```python
from build123d import *

# Parameters (mm, degrees)
F0_W     = 254
F0_H     = 101.6
F0_R     = 9.525
F1_DEPTH = 12.7
F2_R     = 6.35
F3_DEPTH = 12.7
F4_R     = 6.35
F5_W     = 0.9328643791
F5_H     = 1.7582587898
F5_W_2   = 0.0005662441
F5_H_2   = 0.0007078052
F6_DEPTH = 254.001


# Not quite as in the source:
# - a feature of the source that left no trace in its solid (it failed there, or was rolled back) is left out


with BuildPart() as f1:
    # F0 (on Front) → F1 (new body)
    with BuildSketch(Plane.XZ):
        with Locations((143.2877514958, 67.8497503132)):
            Rectangle(F0_W, F0_H)
        with Locations((67.0877514958, 67.8497503132)):
            Circle(F0_R, mode=Mode.SUBTRACT)
        with Locations((219.4877514958, 67.8497503132)):
            Circle(F0_R, mode=Mode.SUBTRACT)
    extrude(amount=F1_DEPTH)

    # F2
    f2_edges = [f1.edges().sort_by_distance(p)[0] for p in [
        (16.287751, -6.35, 118.64975),
        (16.287751, -6.35, 17.04975),
        (270.287751, -6.35, 118.64975),
        (270.287751, -6.35, 17.04975),
    ]]
    fillet(f2_edges, radius=F2_R)

    # F0 (on Front) → F3 (join)
    with BuildSketch(Plane.XZ):
        with Locations((143.2877514958, 67.8497503132)):
            Rectangle(F0_W, F0_H)
        with Locations((67.0877514958, 67.8497503132)):
            Circle(F0_R, mode=Mode.SUBTRACT)
        with Locations((219.4877514958, 67.8497503132)):
            Circle(F0_R, mode=Mode.SUBTRACT)
    extrude(amount=F3_DEPTH)

    # F4
    f4_edges = [f1.edges().sort_by_distance(p)[0] for p in [
        (270.287751, -6.35, 118.64975),
        (16.287751, -6.35, 118.64975),
        (270.287751, -6.35, 17.04975),
        (16.287751, -6.35, 17.04975),
    ]]
    fillet(f4_edges, radius=F4_R)

    # F5 (on face) → F6 (cut, through all)
    with BuildSketch(Plane(origin=(16.2877514958, 0, 0), x_dir=(0, -1, 0), z_dir=(-1, 0, 0))):
        with Locations((6.063854089, 49.9223377556)):
            Rectangle(F5_W, F5_H)
        with Locations((8.4549216554, 49.0087680519)):
            Rectangle(F5_W_2, F5_H_2)
    extrude(amount=-F6_DEPTH, mode=Mode.SUBTRACT)


solid = f1.part
```
The listing builds one solid part. Answer for the finished solid, in the listing's coordinates (mm). Coordinates: 2 decimals unless noted, no trailing zeros. Loops run counter-clockwise (first coordinate to the right, second up) from the corner with the lowest first, then second, coordinate; pieces in that order, holes last. Notation, with made-up numbers: (-9, 46.5) -> (21, 46.5) arc R26 ccw to (21, 81.5) -> close; hole circle Ø10 at (81.5, -27). An arc over 180 degrees is marked (long way). Return JSON: item names as keys, results as strings. Group by question number.
(1) Determine the mould class of faces 1 (the flat face through (16.288, -6, 67)), 2 (the flat face through (142, 0, 69)), 3 (the cylindrical face through (57.572, -6.261, 68.269)) for opening direction X: released by +X, released by -X, zero draft, split by the parting line, or undercut.
(2) A cutting plane is placed at A-A on y = -10.5. Write down the section's boundary in (x, z) (3 decimals).
(3) Find the intervals of material crossed by probe 1 along Z at (x, y) = (123.5, -6.25); probe 2 along Z at (x, y) = (68, -8.25); probe 3 along X at (y, z) = (-1, 71), in increasing order. Write a range as from..to.
(4) Given pin 1 Ø2 at (x, z) = (186.5, 98) entering from +Y, flat-ended and moving along its own axis, determine where the tip first touches the part or whether it passes through.
The answers:
{
 "1": {"face 1": "released by -X", "face 2": "zero draft", "face 3": "undercut"},
 "2": {"outline": "(16.288, 23.4) arc R6.35 ccw to (22.638, 17.05) -> (263.938, 17.05) arc R6.35 ccw to (270.288, 23.4) -> (270.288, 112.3) arc R6.35 ccw to (263.938, 118.65) -> (22.638, 118.65) arc R6.35 ccw to (16.288, 112.3) -> close; hole circle Ø19.05 at (67.088, 67.85); hole circle Ø19.05 at (219.488, 67.85)"},
 "3": {"probe 1": "z = 17.05..49.04, 50.8..118.65", "probe 2": "z = 17.05..58.37, 77.33..118.65", "probe 3": "x = 16.29..58.1, 76.08..210.5, 228.48..270.29"},
 "4": {"pin 1": "stops at y = 0"}
}
